Build history of the part. All positions in model axes, mm. A direction names the side the tool comes from. Give positions to 0.01 mm unless a question says otherwise; leave off trailing zeros. Order: outer loops, then holes, each group sorted by start corner. A loop starts at its lowest first (then second) coordinate and runs counter-clockwise, first axis right, second up. Notation, with made-up numbers: (4.25, 48) -> (20.25, 48) arc R26 cw to (20.25, 70) -> close; hole circle Ø2 at (-20, -8.5). An arc over 180 degrees is marked (long way). One line per question, with ' | ' between items. Start each with the question number.
(1) Pull direction X, two halves, no side cores. Call faces 3 (the face through (-69, 1.588, -1)), 4 (the face through (-61.96, 0.78, 61.49)), 5 (the face through (36.868, 3.779, -57.827)): +X half, -X half, draft (parallel to the pull), parting line (faces both ways), or undercut.
(2) Cut at A-A (z = 0). Give the cut face in (x, y), then the cut area to 3 significant figures.
(3) Which spindle directions (+Z, -Z, +X, -X, +Y, -Y) get a long thin tool onto all of the face, cutting with end or side? Do faces 1 (the face through (63, 3.8, -19.8)), 2 (the face through (62.3, 0.8, -59)). Say none if no direction does.
(4) Cut at C-C (y = 4.5). Give the cut face in (x, z).
(5) Pin check, flat tips, straight feed: pin 1 Ø2 at (x, y) = (29, 5) entering from +Z; pin 2 Ø2 at (x, y) = (-33, 3) entering from +Z; pin 3 Ø6 at (x, z) = (-59.944, -59.944) entering from +Y. Stop position of each tip, or through.
(6) Drill centre lines: L1, parallel to X at y = 3.5, z = 0; L2, parallel to Y at x = 61.5, z = -44; L3, parallel to Z at x = -40.5, y = 3.5. Where is each one in solid material? Low to high. Write a range as from..to.
(7) Cut at B-B (x = 0). Give the cut face in (y, z).
from build123d import *

# Parameters (mm, degrees)
SKETCH1_W           = 152.4
SKETCH1_H           = 152.4
SKETCH1_R           = 63.5
SKETCH1_R_2         = 2.54
BOSS_EXTRUDE1_DEPTH = 1.5875
SKETCH2_R           = 68.58
SKETCH2_R_2         = 66.04
BOSS_EXTRUDE2_DEPTH = 4.445


with BuildPart() as part:
    # Sketch1 → Boss-Extrude1 (new body)
    with BuildSketch(Plane(origin=(0, 0, 0), x_dir=(1, 0, 0), z_dir=(0, 1, 0))):
        Rectangle(SKETCH1_W, SKETCH1_H)
        Circle(SKETCH1_R, mode=Mode.SUBTRACT)
        with Locations((-59.944, 59.944)):
            Circle(SKETCH1_R_2, mode=Mode.SUBTRACT)
        with Locations((59.944, 59.944)):
            Circle(SKETCH1_R_2, mode=Mode.SUBTRACT)
        with Locations((59.944, -59.944)):
            Circle(SKETCH1_R_2, mode=Mode.SUBTRACT)
        with Locations((-59.944, -59.944)):
            Circle(SKETCH1_R_2, mode=Mode.SUBTRACT)
    extrude(amount=BOSS_EXTRUDE1_DEPTH)

    # Sketch2 → Boss-Extrude2 (add)
    with BuildSketch(Plane(origin=(0, 1.5875, 0), x_dir=(1, 0, 0), z_dir=(0, 1, 0))):
        Circle(SKETCH2_R)
        Circle(SKETCH2_R_2, mode=Mode.SUBTRACT)
    extrude(amount=BOSS_EXTRUDE2_DEPTH)


solid = part.part
Result set:
1) face 3: draft | face 4: undercut | face 5: parting line
2) outline: (-76.2, 0) -> (-63.5, 0) -> (-63.5, 1.59) -> (-66.04, 1.59) -> (-66.04, 6.03) -> (-68.58, 6.03) -> (-68.58, 1.59) -> (-76.2, 1.59) -> close; (63.5, 0) -> (76.2, 0) -> (76.2, 1.59) -> (68.58, 1.59) -> (68.58, 6.03) -> (66.04, 6.03) -> (66.04, 1.59) -> (63.5, 1.59) -> close | area: 62.9 mm2
3) face 1: +Y | face 2: +Y, -Y
4) outline: circle Ø137.16 at (0, 0); hole circle Ø132.08 at (0, 0)
5) pin 1: stops at z = 62.6 | pin 2: stops at z = 60.66 | pin 3: stops at y = 1.59
6) L1: x = -68.58..-66.04, 66.04..68.58 | L2: y = 0..1.59 | L3: z = -55.34..-52.16, 52.16..55.34
7) outline: (0, -76.2) -> (1.59, -76.2) -> (1.59, -68.58) -> (6.03, -68.58) -> (6.03, -66.04) -> (1.59, -66.04) -> (1.59, -63.5) -> (0, -63.5) -> close; (0, 63.5) -> (1.59, 63.5) -> (1.59, 66.04) -> (6.03, 66.04) -> (6.03, 68.58) -> (1.59, 68.58) -> (1.59, 76.2) -> (0, 76.2) -> close
